Design review of the part built by this model. Coordinates are the model's own, in mm. A direction names the side the tool comes from. Give positions to 0.01 mm unless a question says otherwise; leave off trailing zeros. Write each loop counter-clockwise with the first axis right and the second up, starting at its lowest first coordinate (ties: lowest second). Pieces come first, ordered by that corner, then holes. Notation, with made-up numbers: (74, 83) - (130, 83) arc R18 ccw to (130, 114) - close; hole circle Ø1 at (13.25, -29.5). An arc over 180 degrees is marked (long way). Write each question's results on one line, items separated by ' | '. Start each with the question number.
from build123d import *

# Parameters (mm, degrees)
SKETCH_W        = 90.5
SKETCH_H        = 62.5
PAD_DEPTH       = 52
SKETCH001_W     = 85.5
SKETCH001_H     = 56.5
POCKET_DEPTH    = 50
SKETCH002_W     = 61
SKETCH002_H     = 3
POCKET001_DEPTH = 52
SKETCH003_W     = 3
SKETCH003_H     = 1.3
SKETCH003_W_2   = 1.3
SKETCH003_H_2   = 57.8
SKETCH003_W_3   = 86.8
SKETCH003_W_4   = 21.5
PAD001_DEPTH    = 2.5
SKETCH004_W     = 2
SKETCH004_H     = 19.95
PAD002_DEPTH    = 2
PAD003_DEPTH    = 2
FILLET_R        = 3
SKETCH005_W     = 10
SKETCH005_H     = 18
POCKET002_DEPTH = 5
FILLET001_R     = 3
SKETCH006_R     = 1.85
POCKET003_DEPTH = 5


with BuildPart() as part:
    # Sketch → Pad (new body)
    with BuildSketch(Plane.XY):
        Rectangle(SKETCH_W, SKETCH_H)
    extrude(amount=PAD_DEPTH)

    # Sketch001 (on Face6 of Pad) → Pocket (cut)
    with BuildSketch(Plane.XY.offset(52)):
        with Locations((0.5, 0)):
            Rectangle(SKETCH001_W, SKETCH001_H)
    extrude(amount=-POCKET_DEPTH, mode=Mode.SUBTRACT)

    # Sketch002 (on Face5 of Pocket) → Pocket001 (cut)
    with BuildSketch(Plane.XY.offset(52)):
        with Locations((-8.75, 29.75)):
            Rectangle(SKETCH002_W, SKETCH002_H)
    extrude(amount=-POCKET001_DEPTH, mode=Mode.SUBTRACT)

    # Sketch003 (on Face4 of Pocket001) → Pad001 (join)
    with BuildSketch(Plane.XY.offset(52)):
        with Locations((-40.75, 28.9)):
            Rectangle(SKETCH003_W, SKETCH003_H)
        with Locations((-42.9, 0.65)):
            Rectangle(SKETCH003_W_2, SKETCH003_H_2)
        with Locations((-0.15, -28.9)):
            Rectangle(SKETCH003_W_3, SKETCH003_H)
        with Locations((32.5, 28.9)):
            Rectangle(SKETCH003_W_4, SKETCH003_H)
    extrude(amount=PAD001_DEPTH)

    # Sketch004 (on Face4 of Pad001) → Pad002 (join)
    with BuildSketch(Plane.XY.offset(52)):
        with Locations((44.25, 15.725)):
            Rectangle(SKETCH004_W, SKETCH004_H)
    extrude(amount=PAD002_DEPTH)

    # Sketch004 (on Face4 of Pad001) → Pad003 (join)
    with BuildSketch(Plane.XY.offset(52)):
        with Locations((44.25, 15.725)):
            Rectangle(SKETCH004_W, SKETCH004_H)
    extrude(amount=PAD003_DEPTH)

    # Fillet
    fillet_edges = [part.edges().sort_by_distance(p)[0] for p in [
        (45.25, 31.25, 26),
        (45.25, -31.25, 26),
        (-45.25, 31.25, 26),
        (-45.25, -31.25, 26),
    ]]
    fillet(fillet_edges, radius=FILLET_R)

    # Sketch005 (on Face6 of Fillet) → Pocket002 (cut)
    with BuildSketch(Plane(origin=(-45.25, 0, 0), x_dir=(0, -1, 0), z_dir=(-1, 0, 0))):
        with Locations((-17.25, 46)):
            Rectangle(SKETCH005_W, SKETCH005_H)
    extrude(amount=-POCKET002_DEPTH, mode=Mode.SUBTRACT)

    # Fillet001
    fillet001_edges = [part.edges().sort_by_distance(p)[0] for p in [
        (-43.75, 22.25, 37),
        (-43.75, 12.25, 37),
    ]]
    fillet(fillet001_edges, radius=FILLET001_R)

    # Sketch006 (on Face1 of Fillet001) → Pocket003 (cut)
    with BuildSketch(Plane(origin=(-45.25, 0, 0), x_dir=(0, -1, 0), z_dir=(-1, 0, 0))):
        with Locations((-14, 12)):
            Circle(SKETCH006_R)
        with Locations((0, 12)):
            Circle(SKETCH006_R)
        with Locations((14, 12)):
            Circle(SKETCH006_R)
    extrude(amount=-POCKET003_DEPTH, mode=Mode.SUBTRACT)


solid = part.part
Q1. Add section D-D on x = 33. State the section outline as (y, z) points.
Q2. For line 1 along X through (y, z) = (25.5, 47); line 2 along Z through (x, y) = (-43.9, 0); line 3 along Y through (x, z) = (37, 29.5), list the stretches that pass through material, from the lowest coordinate up. Write a range as [from, to].
Q3. Add section C-C on z = 12. State the section outline as (x, y) points, plus the area to 3 significant figures.
Q4. Add section A-A on y = 0. State the section outline as (x, z) points.
Q5. The part is to be moulded in two halves that separate along X. For faces 1 (the face through (-39.25, 30, 27)), 2 (the face through (-43.73, 13.11, 37.9)), 3 (the face through (44.39, -30.35, 26.36)), 4 (the face through (-45.25, 0, 26)), say which applies: +X half, -X half, draft (parallel to the pull), parting line (faces both ways), or undercut.
Q6. Insertion check: P1, Ø2, axis at x = 44.5, z = 52.5, coming from the -Y side; P2, Ø2, axis at y = 0.5, z = 54, coming from the -X side; P3, Ø3, axis at x = 34, z = 54, coming from the +Y side. Each pin has a flat end and moves straight along its axis. Give the tip position at first contact, or say it passes through.
Q7. Add section B-B on z = 44. State the section outline as (x, y) points.
Q8. Machinability: for faces 5 (the face through (21.75, 30, 28)), 6 (the face through (-41, 28.25, 28)), 7 (the face through (-43.77, -15.71, 11.29)), 8 (the face through (44, 5.75, 53)), 9 (the face through (-44, 22.25, 47)), which of the approach directions +Z, -Z, +X, -X, +Y, -Y give a long, thin tool a straight path to every point of the face, cutting with its end or side? Answer none if there is none.
Result:
1) outline: (-31.25, 0) - (31.25, 0) - (31.25, 52) - (29.55, 52) - (29.55, 54.5) - (28.25, 54.5) - (28.25, 2) - (-28.25, 2) - (-28.25, 54.5) - (-29.55, 54.5) - (-29.55, 52) - (-31.25, 52) - close
2) line 1: x = [-45.25, -42.25], [43.25, 45.25] | line 2: z = [0, 10.15], [13.85, 52] | line 3: y = [-31.25, -28.25], [28.25, 31.25]
3) outline: (-45.25, -28.25) arc R3 ccw to (-42.25, -31.25) - (42.25, -31.25) arc R3 ccw to (45.25, -28.25) - (45.25, 28.25) arc R3 ccw to (42.25, 31.25) - (21.75, 31.25) - (21.75, 28.25) - (43.25, 28.25) - (43.25, -28.25) - (-42.25, -28.25) - (-42.25, -15.85) - (-45.25, -15.85) - close; (-45.25, -12.15) - (-42.25, -12.15) - (-42.25, -1.85) - (-45.25, -1.85) - close; (-45.25, 1.85) - (-42.25, 1.85) - (-42.25, 12.15) - (-45.25, 12.15) - close; (-45.25, 15.85) - (-42.25, 15.85) - (-42.25, 28.25) - (-39.25, 28.25) - (-39.25, 31.25) - (-42.25, 31.25) arc R3 ccw to (-45.25, 28.25) - close | area: 601 mm²
4) outline: (-45.25, 0) - (45.25, 0) - (45.25, 52) - (43.25, 52) - (43.25, 2) - (-42.25, 2) - (-42.25, 10.15) - (-45.25, 10.15) - close; (-45.25, 13.85) - (-42.25, 13.85) - (-42.25, 54.5) - (-43.55, 54.5) - (-43.55, 52) - (-45.25, 52) - close
5) face 1: undercut | face 2: draft | face 3: +X half | face 4: -X half
6) P1: stops at y = -30.91 | P2: stops at x = -43.55 | P3: stops at y = 29.55
7) outline: (-45.25, -28.25) arc R3 ccw to (-42.25, -31.25) - (42.25, -31.25) arc R3 ccw to (45.25, -28.25) - (45.25, 28.25) arc R3 ccw to (42.25, 31.25) - (21.75, 31.25) - (21.75, 28.25) - (43.25, 28.25) - (43.25, -28.25) - (-42.25, -28.25) - (-42.25, 12.25) - (-45.25, 12.25) - close; (-45.25, 22.25) - (-42.25, 22.25) - (-42.25, 28.25) - (-39.25, 28.25) - (-39.25, 31.25) - (-42.25, 31.25) arc R3 ccw to (-45.25, 28.25) - close
8) face 5: +Z, -Z, +Y | face 6: +Z | face 7: -X | face 8: +Z, +X, -Y | face 9: +Z, -X
